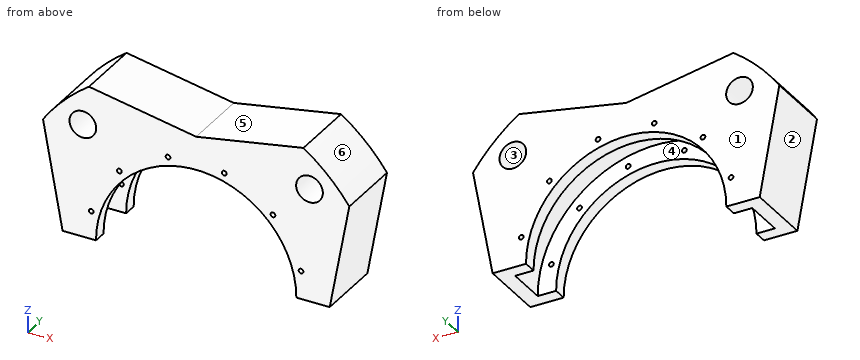
from build123d import *

# Parameters (mm, degrees)
REVOLVE1_ANGLE                 = 180
TAP_DRILL_FOR_4_40_TAP1_D      = 2.2606
CIRPATTERN1_COUNT              = 12
CUT_EXTRUDE1_REACH             = 90.9
SKETCH4_R                      = 1.1303
CUT_EXTRUDE2_REACH             = 90.9
SKETCH6_R                      = 1.1303
CUT_EXTRUDE2_DIRECTION_2_DEPTH = 1.0000001
CUT_EXTRUDE3_REACH             = 33.75
SKETCH7_R                      = 6.35


with BuildPart() as part:
    # Sketch1 → Revolve1 (revolve)
    with BuildSketch(Plane.XY):
        Polygon((56.388, 0), (56.388, 9.525), (47.625, 9.525), (47.625, 15.875), (88.9, 15.875), (88.9, -15.875), (47.625, -15.875), (47.625, -9.525), (56.388, -9.525), align=None)
    revolve(axis=Axis((0, 22.539286723, 0), (0, -1, 0)), revolution_arc=REVOLVE1_ANGLE)

    # Tap Drill for #4-40 Tap1 (through all)
    with Locations(Plane(origin=(49.878671003, 15.875, 13.364949615), x_dir=(0, 0, 1), z_dir=(0, 1, 0))):
        with Locations((0, 0)):
            tap_drill_for_4_40_tap1 = Hole(TAP_DRILL_FOR_4_40_TAP1_D / 2)

    # CirPattern1: Tap Drill for #4-40 Tap1 ×12 about axis, 6 skipped
    cirpattern1_axis = Axis((0, 15.875, 0), (0, 1, 0))
    add([tap_drill_for_4_40_tap1.rotate(cirpattern1_axis, i * 360 / CIRPATTERN1_COUNT) for i in range(1, CIRPATTERN1_COUNT) if i not in (1, 2, 3, 4, 5, 6)], mode=Mode.SUBTRACT)

    # Sketch4 → Cut-Extrude1 (cut, up to next)
    with BuildSketch(Plane(origin=(0, 0, 0), x_dir=(-1, 0, 0), z_dir=(0, 0, -1)), mode=Mode.PRIVATE) as cut_extrude1_sk1:
        with Locations((82.55, 6.35)):
            Circle(SKETCH4_R)
    cut_extrude1_tool1 = extrude(cut_extrude1_sk1.sketch, amount=-CUT_EXTRUDE1_REACH, mode=Mode.PRIVATE) & part.part
    add(cut_extrude1_tool1.solids().sort_by_distance((-82.55, 6.35, 0))[0], mode=Mode.SUBTRACT)
    # Sketch4 → Cut-Extrude1 (cut, up to next)
    with BuildSketch(Plane(origin=(0, 0, 0), x_dir=(-1, 0, 0), z_dir=(0, 0, -1)), mode=Mode.PRIVATE) as cut_extrude1_sk2:
        with Locations((82.55, -6.35)):
            Circle(SKETCH4_R)
    cut_extrude1_tool2 = extrude(cut_extrude1_sk2.sketch, amount=-CUT_EXTRUDE1_REACH, mode=Mode.PRIVATE) & part.part
    add(cut_extrude1_tool2.solids().sort_by_distance((-82.55, -6.35, 0))[0], mode=Mode.SUBTRACT)

    # Sketch6 → Cut-Extrude2 (cut, up to next)
    with BuildSketch(Plane(origin=(0, 0, 0), x_dir=(-1, 0, 0), z_dir=(0, 0, -1)), mode=Mode.PRIVATE) as cut_extrude2_sk1:
        with Locations((-82.55, 6.35)):
            Circle(SKETCH6_R)
    cut_extrude2_tool1 = extrude(cut_extrude2_sk1.sketch, amount=-CUT_EXTRUDE2_REACH, mode=Mode.PRIVATE) & part.part
    add(cut_extrude2_tool1.solids().sort_by_distance((82.55, 6.35, 0))[0], mode=Mode.SUBTRACT)
    # Sketch6 → Cut-Extrude2 (cut, up to next)
    with BuildSketch(Plane(origin=(0, 0, 0), x_dir=(-1, 0, 0), z_dir=(0, 0, -1)), mode=Mode.PRIVATE) as cut_extrude2_sk2:
        with Locations((-82.579243869, -6.35)):
            Circle(SKETCH6_R)
    cut_extrude2_tool2 = extrude(cut_extrude2_sk2.sketch, amount=-CUT_EXTRUDE2_REACH, mode=Mode.PRIVATE) & part.part
    add(cut_extrude2_tool2.solids().sort_by_distance((82.579244, -6.35, 0))[0], mode=Mode.SUBTRACT)

    # Sketch6 → Cut-Extrude2 direction 2 (cut)
    with BuildSketch(Plane(origin=(0, 0, 0), x_dir=(-1, 0, 0), z_dir=(0, 0, -1))):
        with Locations((-82.55, 6.35)):
            Circle(SKETCH6_R)
        with Locations((-82.579243869, -6.35)):
            Circle(SKETCH6_R)
    extrude(amount=CUT_EXTRUDE2_DIRECTION_2_DEPTH, mode=Mode.SUBTRACT)

    # Sketch7 → Cut-Extrude3 (cut, up to next)
    with BuildSketch(Plane(origin=(0, 15.875, 0), x_dir=(1, 0, 0), z_dir=(0, 1, 0)), mode=Mode.PRIVATE) as cut_extrude3_sk1:
        with Locations((53.881536726, -53.881536726)):
            Circle(SKETCH7_R)
    cut_extrude3_tool1 = extrude(cut_extrude3_sk1.sketch, amount=-CUT_EXTRUDE3_REACH, mode=Mode.PRIVATE) & part.part
    add(cut_extrude3_tool1.solids().sort_by_distance((53.881537, 15.875, 53.881537))[0], mode=Mode.SUBTRACT)
    # Sketch7 → Cut-Extrude3 (cut, up to next)
    with BuildSketch(Plane(origin=(0, 15.875, 0), x_dir=(1, 0, 0), z_dir=(0, 1, 0)), mode=Mode.PRIVATE) as cut_extrude3_sk2:
        with Locations((-53.881536726, -53.881536726)):
            Circle(SKETCH7_R)
    cut_extrude3_tool2 = extrude(cut_extrude3_sk2.sketch, amount=-CUT_EXTRUDE3_REACH, mode=Mode.PRIVATE) & part.part
    add(cut_extrude3_tool2.solids().sort_by_distance((-53.881537, 15.875, 53.881537))[0], mode=Mode.SUBTRACT)
    # Sketch7 → Cut-Extrude3 (cut, up to next)
    with BuildSketch(Plane(origin=(0, 15.875, 0), x_dir=(1, 0, 0), z_dir=(0, 1, 0)), mode=Mode.PRIVATE) as cut_extrude3_sk3:
        with BuildLine():
            ThreePointArc((-50.990945192, -72.822616737), (0, -88.9), (50.990945192, -72.822616737))
            Line((50.990945192, -72.822616737), (0, -63.5))
            Line((0, -63.5), (-50.990945192, -72.822616737))
        make_face()
    cut_extrude3_tool3 = extrude(cut_extrude3_sk3.sketch, amount=-CUT_EXTRUDE3_REACH, mode=Mode.PRIVATE) & part.part
    add(cut_extrude3_tool3.solids().sort_by_distance((0, 15.875, 76.438451))[0], mode=Mode.SUBTRACT)
    # Sketch7 → Cut-Extrude3 (cut, up to next)
    with BuildSketch(Plane(origin=(0, 15.875, 0), x_dir=(1, 0, 0), z_dir=(0, 1, 0)), mode=Mode.PRIVATE) as cut_extrude3_sk4:
        with BuildLine():
            Line((63.5, 0), (72.822616737, -50.990945192))
            ThreePointArc((72.822616737, -50.990945192), (84.785436922, -26.732745576), (88.9, 0))
            Line((88.9, 0), (63.5, 0))
        make_face()
    cut_extrude3_tool4 = extrude(cut_extrude3_sk4.sketch, amount=-CUT_EXTRUDE3_REACH, mode=Mode.PRIVATE) & part.part
    add(cut_extrude3_tool4.solids().sort_by_distance((76.438451, 15.875, 18.664198))[0], mode=Mode.SUBTRACT)
    # Sketch7 → Cut-Extrude3 (cut, up to next)
    with BuildSketch(Plane(origin=(0, 15.875, 0), x_dir=(1, 0, 0), z_dir=(0, 1, 0)), mode=Mode.PRIVATE) as cut_extrude3_sk5:
        with BuildLine():
            Line((-72.822616737, -50.990945192), (-63.5, 0))
            Line((-63.5, 0), (-88.9, 0))
            ThreePointArc((-88.9, 0), (-84.785436922, -26.732745576), (-72.822616737, -50.990945192))
        make_face()
    cut_extrude3_tool5 = extrude(cut_extrude3_sk5.sketch, amount=-CUT_EXTRUDE3_REACH, mode=Mode.PRIVATE) & part.part
    add(cut_extrude3_tool5.solids().sort_by_distance((-76.438451, 15.875, 18.664198))[0], mode=Mode.SUBTRACT)


solid = part.part
CAD build for the part. Positions are in the model's coordinates, mm. Face numbers are marked on the shaded views. A direction names the side the tool comes from. Give positions to 0.01 mm unless a question says otherwise; leave off trailing zeros. Order: outer loops, then holes, each group sorted by start corner. A loop starts at its lowest first (then second) coordinate and runs counter-clockwise, first axis right, second up. Notation, with made-up numbers: (78.5, 8.5) - (97.5, 8.5) arc R13 ccw to (97.5, 17.5) - close; hole circle Ø3 at (66.5, 46.5). An arc over 180 degrees is marked (long way). Answer in a Markdown table with one row per item.
1. Saw through at B-B, the plane y = -13. Count the separate pieces of the cut face and the enclosed holes in it, plus the area to 3 significant figures.
Data:
| item | result |
|---|---|
| separate pieces | 1 |
| enclosed holes | 8 |
| area | 5,390 mm² |
2. Tool access for the marked faces 4, 5 and 6: list every direction of +Z, -Z, +X, -X, +Y, -Y with a clear straight run to the whole face (end or side of a thin tool).
Data:
| item | result |
|---|---|
| face 4 | -Z |
| face 5 | +Z, +Y, -Y |
| face 6 | +Z, +X, +Y, -Y |
3. Flat gauge pins, fed straight in: pin 1 (1.4 mm diameter, centred on x = 13.36, z = 49.88, fed in from -Y); pin 2 (4 mm diameter, centred on x = 54, y = 0.5, fed in from +Z); pin 3 (5 mm diameter, centred on x = 29.5, y = -8, fed in from -Z); pin 4 (2 mm diameter, centred on y = -11, z = 11.5, fed in from +X). Where does each tip first touch, or does it go through?
Data:
| item | result |
|---|---|
| pin 1 | passes through |
| pin 2 | stops at z = 72.11 |
| pin 3 | stops at z = 35.74 |
| pin 4 | stops at x = 65.79 |
4. Probe probe 1 along Y at (x, z) = (-15.5, 51) (3 decimals); probe 2 along X at (y, z) = (7, 57); probe 3 along X at (y, z) = (-8.5, 50). List the from-to ranges inside material, lowest first. Write a range as [from, to].
Data:
| item | result |
|---|---|
| probe 1 | y = [-15.875, -9.525], [9.525, 15.875] |
| probe 2 | x = [-68.22, -59.41], [-48.35, 48.35], [59.41, 68.22] |
| probe 3 | x = [-72.64, -58.91], [-48.86, -26.07], [26.07, 48.86], [58.91, 72.64] |
5. Pull direction X, two halves, no side cores. Call the marked faces 1, 2 and 3: pulls with the +X half, pulls with the -X half, needs draft (parallel to the pull), parting line crosses it, or undercut.
Data:
| item | result |
|---|---|
| face 1 | needs draft |
| face 2 | pulls with the -X half |
| face 3 | undercut |
6. Saw through at D-D, the plane x = 18. Give the cut face in (y, z) (3 decimals), plus the area to 3 significant figures.
Data:
| item | result |
|---|---|
| outline | (-15.875, 44.092) - (-9.525, 44.092) - (-9.525, 53.438) - (9.525, 53.438) - (9.525, 44.092) - (15.875, 44.092) - (15.875, 66.791) - (-15.875, 66.791) - close |
| area | 543 mm² |
7. Saw through at A-A, the plane z = 19. Give the cut face in (x, y) (3 decimals), plus the area to 3 significant figures.
Data:
| item | result |
|---|---|
| outline | (-66.974, -15.875) - (-43.671, -15.875) - (-43.671, -9.525) - (-53.091, -9.525) - (-53.091, 9.525) - (-43.671, 9.525) - (-43.671, 15.875) - (-66.974, 15.875) - close; (43.671, -15.875) - (66.974, -15.875) - (66.974, 15.875) - (43.671, 15.875) - (43.671, 9.525) - (53.091, 9.525) - (53.091, -9.525) - (43.671, -9.525) - close |
| area | 1,120 mm² |
8. Saw through at C-C, the plane y = 2. Give the cut face in (x, z), plus the area to 3 significant figures.
Data:
| item | result |
|---|---|
| outline | (-72.82, 50.99) - (-63.5, 0) - (-56.39, 0) arc R56.39 cw to (56.39, 0) - (63.5, 0) - (72.82, 50.99) arc R88.9 ccw to (50.99, 72.82) - (0, 63.5) - (-50.99, 72.82) arc R88.9 ccw to start; hole circle Ø12.7 at (-53.88, 53.88); hole circle Ø12.7 at (53.88, 53.88) |
| area | 3,990 mm² |
